For this review, take the finished solid that the model builds, in its own axes (mm). Round coordinates to 2 decimals unless told otherwise and drop trailing zeros. Loops run counter-clockwise (first coordinate to the right, second up) from the corner with the lowest first, then second, coordinate; pieces in that order, holes last.
1) Take a section at B-B (y = 1150). State the section outline as (x, z) points, then the cut area to 3 significant figures.
2) Mouldability with a two-part tool opening along Y and no side actions: class faces 1 (the flat face through (-1, -18, -100)), 2 (the flat face through (-1, -1250, 1)), 3 (the cylindrical face through (-23.07, 1105.64, -1.4)) as pulls with the +Y half, pulls with the -Y half, needs draft (parallel to the pull), parting line crosses it, or undercut.
3) Wall thickness on L1, parallel to Y at x = -3, z = 47.5; L2, parallel to Y at x = 0, z = -3: over which ranges is each line inside the solid? List them lowest first.
4) Take a section at C-C (z = 35). State the section outline as (x, y) points.
5) Take a section at A-A (x = 0). State the section outline as (y, z) points, then the cut area to 3 significant figures.
```python
from build123d import *

# Parameters (mm, degrees)
F0_W     = 200
F0_H     = 200
F1_DEPTH = 1250
F3_D     = 100
F3_DEPTH = 200


with BuildPart() as f1:
    # F0 (on Front) → F1 (new body, symmetric)
    with BuildSketch(Plane.XZ):
        Rectangle(F0_W, F0_H)
    extrude(amount=F1_DEPTH, both=True)

    # F3
    with Locations(Plane.XY.offset(100)):
        with Locations((0, 1150)):
            Hole(F3_D / 2, depth=F3_DEPTH)


solid = f1.part
```
Response:
1. outline: (-100, -100) - (-50, -100) - (-50, 100) - (-100, 100) - close; (50, -100) - (100, -100) - (100, 100) - (50, 100) - close
1. area: 20,000 mm2
2. face 1: needs draft
2. face 2: pulls with the -Y half
2. face 3: undercut
3. L1: y = -1250 to 1100.09, 1199.91 to 1250
3. L2: y = -1250 to 1100, 1200 to 1250
4. outline: (-100, -1250) - (100, -1250) - (100, 1250) - (-100, 1250) - close; hole circle Ø100 at (0, 1150)
5. outline: (-1250, -100) - (1100, -100) - (1100, 100) - (-1250, 100) - close; (1200, -100) - (1250, -100) - (1250, 100) - (1200, 100) - close
5. area: 480,000 mm2
